Check sheet for the modelled part. Datum: model origin and axes. Units: mm. Round coordinates to 2 decimals unless told otherwise and drop trailing zeros. Write each loop counter-clockwise with the first axis right and the second up, starting at its lowest first coordinate (ties: lowest second). Pieces come first, ordered by that corner, then holes.
Item 1: Release check for a two-part mould opening along X. For faces 1 (the cylindrical face through (18.3, -15.1, -1)), 2 (the flat face through (0, -30, -1)), 3 (the flat face through (30, -30, 0)) record: pulls with the +X half, pulls with the -X half, needs draft (parallel to the pull), parting line crosses it, or undercut.
Item 2: Section check C-C, the plane z = -0.55. Record the cut outline in (x, y), plus the area to 3 significant figures.
Item 3: Depth check by flat-ended pin: pin 1 (1 mm diameter, centred on y = -12, z = -0.5, fed in from +X). Enter the tip coordinate at first touch or a pass-through.
Item 4: Section check B-B, the plane x = 15. Record the cut outline in (y, z).
Item 5: Section check A-A, the plane y = -15. Record the cut outline in (x, z), plus the area to 3 significant figures.
Item 6: Material ranges on line 1 along Y through (x, z) = (15, -1.25); line 2 along X through (y, z) = (-45, -0.7); line 3 along X through (y, z) = (-46, -0.25), recorded low to high.
Item 7: Section check D-D, the plane x = 45. Record the cut outline in (y, z).
from build123d import *

# Parameters (mm, degrees)
EXTRUDE_1_DEPTH   = 2
HOLE_WIZARD_M61_D = 6.6
CHAMFER_1_SIZE    = 2


with BuildPart() as part:
    # Эскиз1 → Бобышка-Вытянуть1 (new body)
    with BuildSketch(Plane(origin=(0, 0, 0), x_dir=(1, 0, 0), z_dir=(0, 0, -1))):
        Polygon((0, 0), (0, 60), (60, 60), (60, 30), (30, 0), align=None)
    extrude(amount=EXTRUDE_1_DEPTH)

    # Отверстие с зазором M61 (through all)
    with Locations(Plane(origin=(0, 0, -2), x_dir=(1, 0, 0), z_dir=(0, 0, -1))):
        with Locations((15, 45), (15, 15), (45, 45)):
            Hole(HOLE_WIZARD_M61_D / 2)

    # Фаска1
    chamfer_1_edges = [part.edges().sort_by_distance(p)[0] for p in [
        (0, 0, -1),
        (0, -60, -1),
        (60, -60, -1),
    ]]
    chamfer(chamfer_1_edges, length=CHAMFER_1_SIZE)


solid = part.part
Values found:
1. face 1: undercut
1. face 2: pulls with the -X half
1. face 3: needs draft
2. outline: (0, -58) - (2, -60) - (58, -60) - (60, -58) - (60, -30) - (30, 0) - (2, 0) - (0, -2) - close; hole circle Ø6.6 at (15, -45); hole circle Ø6.6 at (15, -15); hole circle Ø6.6 at (45, -45)
2. area: 3,040 mm2
3. pin 1: stops at x = 42.5
4. outline: (-60, -2) - (-48.3, -2) - (-48.3, 0) - (-60, 0) - close; (-41.7, -2) - (-18.3, -2) - (-18.3, 0) - (-41.7, 0) - close; (-11.7, -2) - (0, -2) - (0, 0) - (-11.7, 0) - close
5. outline: (0, -2) - (11.7, -2) - (11.7, 0) - (0, 0) - close; (18.3, -2) - (45, -2) - (45, 0) - (18.3, 0) - close
5. area: 76.8 mm2
6. line 1: y = -60 to -48.3, -41.7 to -18.3, -11.7 to 0
6. line 2: x = 0 to 11.7, 18.3 to 41.7, 48.3 to 60
6. line 3: x = 0 to 11.86, 18.14 to 41.86, 48.14 to 60
7. outline: (-60, -2) - (-48.3, -2) - (-48.3, 0) - (-60, 0) - close; (-41.7, -2) - (-15, -2) - (-15, 0) - (-41.7, 0) - close
